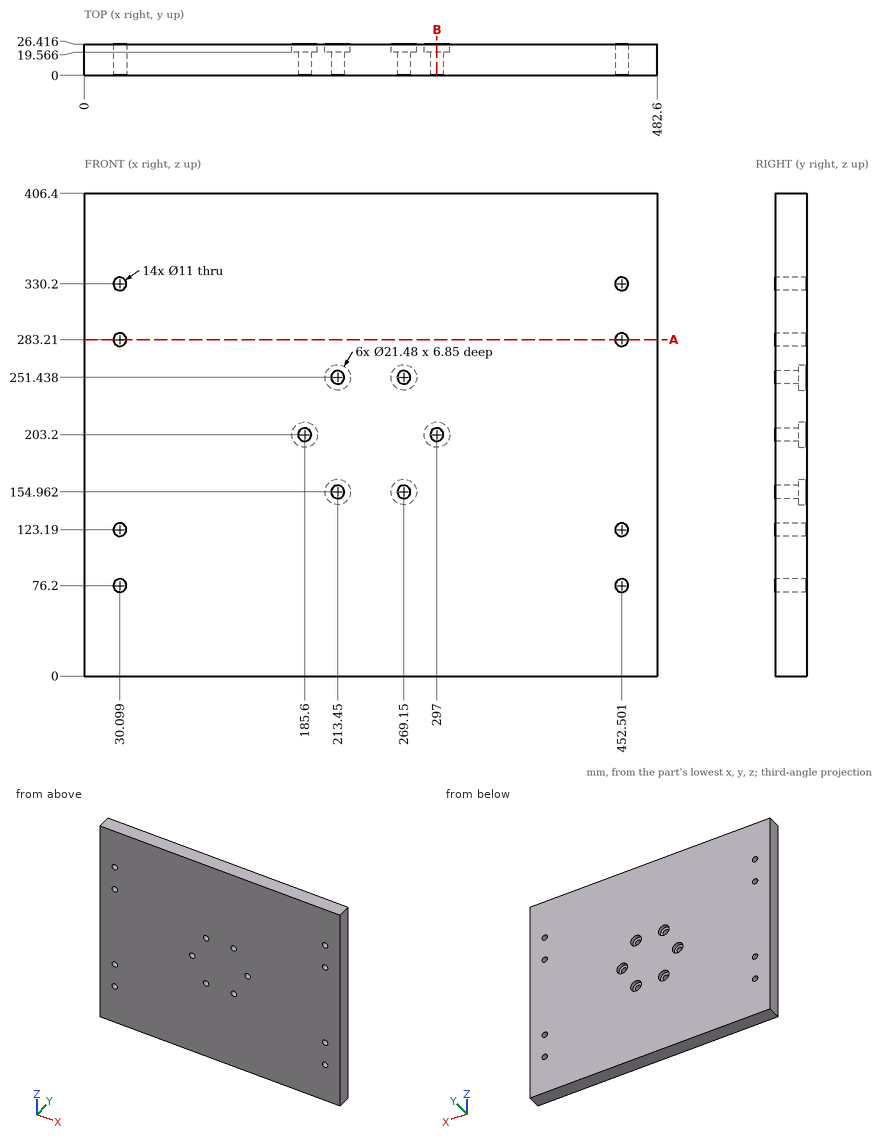
Here's the drawing with two shaded views (mm, measured from the low corner). I have some questions. Give positions to 0.01 mm unless a question says otherwise; leave off trailing zeros. Loops run counter-clockwise (first coordinate to the right, second up) from the corner with the lowest first, then second, coordinate; pieces in that order, holes last. Notation, with made-up numbers: M 47.5,-22 L 99.5,-22 A17 cw 99.5,6 Z; hole C -30,3.5 d10. An arc over 180 degrees is marked long. One line per item, written item: value. Start each with the question number.
1) If we section it at B-B, the plane x = 297: Write out the boundary of the cut face in (y, z).
2) I'm going to push a flat-ended pin straight in: pin 1 (13 mm diameter, centred on x = 297, z = 203.2, fed in from +Y). Where does the tip first touch, or does it pass through?
3) If I drill on line 1 (X direction, y = 7.25, z = 330.2); line 2 (Z direction, x = 213.45, y = 21.5); line 3 (Z direction, x = 274, y = 24.5) (1 decimal), over which ranges is the centre line in solid material (lowest first)? Write a range as [from, to].
4) If we section it at A-A, the plane z = 283.21: Write out the boundary of the cut face in (x, y), and give its area (3 significant figures).
Completed:
1. outline: M 0,0 L 26.42,0 L 26.42,192.46 L 19.57,192.46 L 19.57,197.7 L 0,197.7 Z; M 0,208.7 L 19.57,208.7 L 19.57,213.94 L 26.42,213.94 L 26.42,406.4 L 0,406.4 Z
2. pin 1: stops at y = 19.57
3. line 1: x = [0, 24.6], [35.6, 447], [458, 482.6]
3. line 2: z = [0, 144.22], [165.7, 240.7], [262.18, 406.4]
3. line 3: z = [0, 145.4], [164.5, 241.9], [261, 406.4]
4. outline: M 0,0 L 24.6,0 L 24.6,26.42 L 0,26.42 Z; M 35.6,0 L 447,0 L 447,26.42 L 35.6,26.42 Z; M 458,0 L 482.6,0 L 482.6,26.42 L 458,26.42 Z
4. area: 12,200 mm^2
